The model under review builds one solid part; all positions refer to its coordinate system, in mm. Face numbers are marked on the shaded views. Coordinates: 2 decimals unless noted, no trailing zeros. Write each loop counter-clockwise with the first axis right and the second up, starting at its lowest first coordinate (ties: lowest second). Pieces come first, ordered by that corner, then holes. Notation, with made-up numbers: (51, 60.5) - (102, 60.5) arc R21 ccw to (102, 96.5) - close; hole circle Ø5 at (-20, 82). An arc over 180 degrees is marked (long way). Put each result on its own line as item: value. Start each with the question number.
Item 1: Consider section D-D on z = 15. State how many separate pieces and enclosed holes the cut face has, then the cut area to 3 significant figures.
Item 2: Consider section A-A on x = 0. Give the boundary of the cut face in (y, z), then the cut area to 3 significant figures.
Item 3: Consider section B-B on z = 0. Give the boundary of the cut face in (x, y), then the cut area to 3 significant figures.
Item 4: Consider section C-C on y = 0.75. Give the boundary of the cut face in (x, z).
Item 5: To check wall thickness, follow L1, parallel to Z at x = 0, y = 0.9; L2, parallel to Z at x = 25, y = 0.5; L3, parallel to Z at x = 0, y = 0.95. State the ranges of each line that lie inside material, in increasing order. Write a range as [from, to].
Item 6: For pin 1 (1.5 mm diameter, centred on x = -19.5, z = 8.5, fed in from -Y); pin 2 (1.5 mm diameter, centred on x = 27, y = 3.5, fed in from +Z), all flat-tipped, find the tip position at first contact; note any pin that passes through.
Item 7: Mouldability with a two-part tool opening along X and no side actions: class the marked faces 1, 2 and 3 as pulls with the +X half, pulls with the -X half, needs draft (parallel to the pull), parting line crosses it, or undercut.
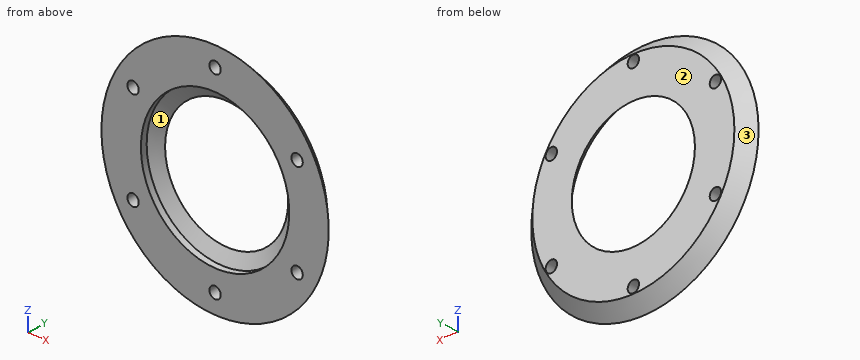
Autodesk Inventor part; units mm, degrees
ref_plane "YZ Plane" through (0, 0, 0) normal (1, 0, 0) x (0, 1, 0)
ref_plane "XZ Plane" through (0, 0, 0) normal (0, 1, 0) x (-1, 0, 0)
ref_plane "XY Plane" through (0, 0, 0) normal (0, 0, 1) x (1, 0, 0)
sketch "Sketch1" plane through (0, 0, 0) normal (0, 0, 1) x (1, 0, 0)
  line L0 (0, 0) -> (0, 4)
  line L1 (-23.5, 0) -> (-36, 0)
  line L2 (-36, 0) -> (-32, 4)
  line L3 (-32, 4) -> (-19.5, 4)
  line L4 (-19.5, 4) -> (-23.5, 2)
  line L5 (-23.5, 2) -> (-23.5, 0)
  point P0 (-29.75, 0)
  dimension "d0" = 47
  dimension "d1" = 12.5
  dimension "d2" = 2
  dimension "d3" = 4
  dimension "d4" = 2
  dimension "d5" = 45
revolve "Revolution1" add sketch "Sketch1" angle 360 about axis through (0, 0, 0) along (0, 1, 0)
sketch "Sketch2" plane through (0, 4, 0) normal (0, 1, 0) x (1, 0, 0)
  circle A0 centre (0, 0) radius 23.5 construction
  circle A1 centre (0, 0) radius 36 construction
  point P0 (0, -30)
  point P1 (25.9808, -15)
  point P2 (25.9808, 15)
  point P3 (0, 30)
  point P4 (-25.9808, 15)
  point P5 (-25.9808, -15)
  dimension "d10" = 360
  dimension "d19" = 30
hole "Hole1" at (0, 4, 30) at (25.9808, 4, 15) at (25.9808, 4, -15) at (0, 4, -30) at (-25.9808, 4, -15) at (-25.9808, 4, 15) direction (0, -1, 0) diameter 3.6 end through all
properties part number "Ring_New"
Report:
1. separate pieces: 4
1. enclosed holes: 0
1. area: 81.5 mm²
2. outline: (0, -36) - (4, -32) - (4, -31.8) - (0, -31.8) - close; (0, -28.2) - (4, -28.2) - (4, -19.5) - (2, -23.5) - (0, -23.5) - close; (0, 23.5) - (2, 23.5) - (4, 19.5) - (4, 28.2) - (0, 28.2) - close; (0, 31.8) - (4, 31.8) - (4, 32) - (0, 36) - close
2. area: 63.2 mm²
3. outline: (-36, 0) - (-23.5, 0) - (-23.5, 2) - (-19.5, 4) - (-32, 4) - close; (19.5, 4) - (23.5, 2) - (23.5, 0) - (36, 0) - (32, 4) - close
3. area: 92.0 mm²
4. outline: circle Ø70.5 at (0, 0); hole circle Ø3.6 at (-25.98, -15); hole circle Ø3.6 at (-25.98, 15); hole circle Ø47 at (0, 0); hole circle Ø3.6 at (0, -30); hole circle Ø3.6 at (0, 30); hole circle Ø3.6 at (25.98, -15); hole circle Ø3.6 at (25.98, 15)
5. L1: [-35.1, -31.8], [-28.2, -23.5], [23.5, 28.2], [31.8, 35.1]
5. L2: [-25.2, -16.51], [-13.49, 13.49], [16.51, 25.2]
5. L3: [-35.05, -31.8], [-28.2, -23.5], [23.5, 28.2], [31.8, 35.05]
6. pin 1: y = 2.74
6. pin 2: z = 19.77
7. face 1: undercut
7. face 2: needs draft
7. face 3: parting line crosses it
